```python
from build123d import *

# Parameters (mm, degrees)
SKETCH5_R           = 23.5
SKETCH5_R_2         = 21.5
BOSS_EXTRUDE3_DEPTH = 19
SKETCH6_R           = 1.5
BOSS_EXTRUDE4_DEPTH = 3
CIRPATTERN1_COUNT   = 4
FILLET1_R           = 4
CUT_EXTRUDE1_DEPTH  = 15
CIRPATTERN2_COUNT   = 4
CUT_EXTRUDE2_DEPTH  = 1.5
CIRPATTERN3_COUNT   = 4
FILLET2_R           = 1
FILLET3_R           = 1
CUT_EXTRUDE3_START  = -0.192276
SKETCH9_R           = 0.5
CUT_EXTRUDE3_DEPTH  = 2.005815
CIRPATTERN4_COUNT   = 4
SKETCH10_R          = 2.55
CUT_EXTRUDE4_DEPTH  = 2
CIRPATTERN5_COUNT   = 4
SKETCH11_W          = 4.1
SKETCH11_H          = 10
CUT_EXTRUDE5_DEPTH  = 2


with BuildPart() as part:
    # Sketch5 → Boss-Extrude3 (new body)
    with BuildSketch(Plane(origin=(0, 0, 0), x_dir=(1, 0, 0), z_dir=(0, 1, 0))):
        Circle(SKETCH5_R)
        Circle(SKETCH5_R_2, mode=Mode.SUBTRACT)
    extrude(amount=BOSS_EXTRUDE3_DEPTH)

    # Sketch6 → Boss-Extrude4 (add)
    with BuildSketch(Plane(origin=(0, 19, 0), x_dir=(1, 0, 0), z_dir=(0, 1, 0))):
        with BuildLine():
            Line((-3, 0), (-3, 21.289668856))
            ThreePointArc((-3, 21.289668856), (0, 21.5), (3, 21.289668856))
            Line((3, 21.289668856), (3, 0))
            Line((3, 0), (-3, 0))
        make_face()
        with Locations((0, 14)):
            Circle(SKETCH6_R, mode=Mode.SUBTRACT)
    boss_extrude4 = extrude(amount=-BOSS_EXTRUDE4_DEPTH)

    # CirPattern1: Boss-Extrude4 ×4 about axis
    cirpattern1_axis = Axis((0, 0, 0), (0, 1, 0))
    for i in range(1, CIRPATTERN1_COUNT):
        add(boss_extrude4.rotate(cirpattern1_axis, i * 360 / CIRPATTERN1_COUNT))

    # Fillet1
    fillet1_edges = [part.edges().sort_by_distance(p)[0] for p in [
        (-3, 17.5, -21.289668856),
        (3, 17.5, -21.289668856),
        (-21.289668856, 17.5, -3),
        (-21.289668856, 17.5, 3),
        (3, 17.5, 21.289668856),
        (-3, 17.5, 21.289668856),
        (21.289668856, 17.5, -3),
        (21.289668856, 17.5, 3),
    ]]
    fillet(fillet1_edges, radius=FILLET1_R)

    # Sketch7 → Cut-Extrude1 (cut)
    with BuildSketch(Plane(origin=(0, 19, 0), x_dir=(1, 0, 0), z_dir=(0, 1, 0))):
        Polygon((21.341935675, 17.099294988), (16.134723728, 11.892083041), (11.892083041, 16.134723728), (17.099294988, 21.341935675), align=None)
    cut_extrude1 = extrude(amount=-CUT_EXTRUDE1_DEPTH, mode=Mode.SUBTRACT)

    # CirPattern2: Cut-Extrude1 ×4 about axis
    cirpattern2_axis = Axis((0, 0, 0), (0, 1, 0))
    for i in range(1, CIRPATTERN2_COUNT):
        add(cut_extrude1.rotate(cirpattern2_axis, i * 360 / CIRPATTERN2_COUNT), mode=Mode.SUBTRACT)

    # Sketch8 → Cut-Extrude2 (cut)
    with BuildSketch(Plane(origin=(0, 19, 0), x_dir=(1, 0, 0), z_dir=(0, 1, 0))):
        Polygon((-12.859793573, 21.345074947), (-7.348880887, 15.834162262), (-15.834162262, 7.348880887), (-21.345074947, 12.859793573), align=None)
    cut_extrude2 = extrude(amount=-CUT_EXTRUDE2_DEPTH, mode=Mode.SUBTRACT)

    # CirPattern3: Cut-Extrude2 ×4 about axis
    cirpattern3_axis = Axis((0, 0, 0), (0, 1, 0))
    for i in range(1, CIRPATTERN3_COUNT):
        add(cut_extrude2.rotate(cirpattern3_axis, i * 360 / CIRPATTERN3_COUNT), mode=Mode.SUBTRACT)

    # Fillet2
    fillet2_edges = [part.edges().sort_by_distance(p)[0] for p in [
        (-23.5, 19, 0),
        (0, 19, -23.5),
        (22.688205944, 19, -6.123341492),
        (0, 19, 23.5),
    ]]
    fillet(fillet2_edges, radius=FILLET2_R)

    # Fillet3
    fillet3_edges = [part.edges().sort_by_distance(p)[0] for p in [
        (-23.5, 0, 0),
    ]]
    fillet(fillet3_edges, radius=FILLET3_R)

    # Sketch9 → Cut-Extrude3 (cut)
    with BuildSketch(Plane(origin=(-16.481049724, 0, 16.481049724), x_dir=(-0.707106781, 0, -0.707106781), z_dir=(0.707106781, 0, -0.707106781)).offset(CUT_EXTRUDE3_START)):
        with Locations((0, 2)):
            Circle(SKETCH9_R)
    cut_extrude3 = extrude(amount=CUT_EXTRUDE3_DEPTH, mode=Mode.SUBTRACT)

    # CirPattern4: Cut-Extrude3 ×4 about axis
    cirpattern4_axis = Axis((0, 19, 0), (0, -1, 0))
    for i in range(1, CIRPATTERN4_COUNT):
        add(cut_extrude3.rotate(cirpattern4_axis, i * 360 / CIRPATTERN4_COUNT), mode=Mode.SUBTRACT)

    # Sketch10 → Cut-Extrude4 (cut)
    with BuildSketch(Plane(origin=(0, 19, 0), x_dir=(1, 0, 0), z_dir=(0, 1, 0))):
        with Locations((0, 20)):
            Circle(SKETCH10_R)
    cut_extrude4 = extrude(amount=-CUT_EXTRUDE4_DEPTH, mode=Mode.SUBTRACT)

    # CirPattern5: Cut-Extrude4 ×4 about axis
    cirpattern5_axis = Axis((0, 0, 0), (0, 1, 0))
    for i in range(1, CIRPATTERN5_COUNT):
        add(cut_extrude4.rotate(cirpattern5_axis, i * 360 / CIRPATTERN5_COUNT), mode=Mode.SUBTRACT)

    # Sketch11 → Cut-Extrude5 (cut)
    with BuildSketch(Plane(origin=(0, 19, 0), x_dir=(1, 0, 0), z_dir=(0, 1, 0))):
        with Locations((0, -3.45)):
            Rectangle(SKETCH11_W, SKETCH11_H)
    extrude(amount=-CUT_EXTRUDE5_DEPTH, mode=Mode.SUBTRACT)


solid = part.part
```
Verification items for the finished model (mm, model axes). A direction names the side the tool comes from. Coordinates: 2 decimals unless noted, no trailing zeros. Order: outer loops, then holes, each group sorted by start corner. A loop starts at its lowest first (then second) coordinate and runs counter-clockwise, first axis right, second up. Notation, with made-up numbers: (-22, -22) -> (3, -22) arc R14 cw to (3, 0) -> close; hole circle Ø7 at (-12.75, 63.25). An arc over 180 degrees is marked (long way). Put each result on its own line as item: value. Start each with the question number.
1) Material ranges on L1, parallel to Z at x = 0, y = 17.2; L2, parallel to Z at x = -2, y = 18.25; L3, parallel to Z at x = -14, y = 17.8, recorded low to high.
2) Cross-section at A-A (y = 10.75). Enter the section's corners in (x, z).
3) Release check for a two-part mould opening along Y. For faces 1 (the flat face through (0, 16, 0)), 2 (the cylindrical face through (-16.11, 2.42, 15.73)), 3 (the flat face through (-20, 17, 0)), 4 (the flat face through (-11.08, 18.26, 19.565)) record: pulls with the +Y half, pulls with the -Y half, needs draft (parallel to the pull), parting line crosses it, or undercut.
4) Tool access check on faces 5 (the flat face through (10, 18, 3)), 6 (the flat face through (13.66, 10.84, 17.9)), 7 (the cylindrical face through (17.74, 18.01, 1.18)), 8 (the flat face through (-17.9, 10.84, 13.66)). Record the directions out of +Z, -Z, +X, -X, +Y, -Y that give a thin tool (end or side, any length) a straight path to the whole face; none if there is none.
5) Cross-section at B-B (x = 5). State how many separate pieces and enclosed holes the cut face has, plus the area to 3 significant figures.
6) Go/stop test with flat-tipped pins: pin 1 (2.5 mm diameter, centred on x = -18, z = 13, fed in from +Y); pin 2 (1.8 mm diameter, centred on x = -14, z = 0, fed in from -Y); pin 3 (6 mm diameter, centred on y = 8, z = -15, fed in from +X); pin 4 (2.5 mm diameter, centred on y = 17, z = -10.5, fed in from -X). Record where each tip stops, or that it passes through.
Geometry check:
1. L1: z = -23.5 to -22.55, -17.45 to -15.5, -12.5 to -1.55, 8.45 to 12.5, 15.5 to 17.45, 22.55 to 23.5
1. L2: z = -23.38 to -21.58, -18.42 to -1.55, 8.45 to 18.42, 21.58 to 23.38
1. L3: z = -3 to -1.5, 1.5 to 3
2. outline: (-18.6, -14.36) -> (-17.18, -12.93) arc R21.5 cw to (-17.18, 12.93) -> (-18.6, 14.36) arc R23.5 ccw to start; (-14.36, -18.6) arc R23.5 ccw to (14.36, -18.6) -> (12.93, -17.18) arc R21.5 cw to (-12.93, -17.18) -> close; (-14.36, 18.6) -> (-12.93, 17.18) arc R21.5 cw to (12.93, 17.18) -> (14.36, 18.6) arc R23.5 ccw to start; (17.18, -12.93) -> (18.6, -14.36) arc R23.5 ccw to (18.6, 14.36) -> (17.18, 12.93) arc R21.5 cw to start
3. face 1: pulls with the -Y half
3. face 2: undercut
3. face 3: pulls with the +Y half
3. face 4: needs draft
4. face 5: +Y, -Y
4. face 6: +X, +Y
4. face 7: +Y
4. face 8: +Z, +Y
5. separate pieces: 3
5. enclosed holes: 0
5. area: 104 mm^2
6. pin 1: stops at y = 17.5
6. pin 2: passes through
6. pin 3: stops at x = 20.21
6. pin 4: stops at x = -21.6
